Check sheet for the modelled part. Datum: model origin and axes. Units: mm. A direction names the side the tool comes from. Coordinates: 2 decimals unless noted, no trailing zeros. Order: outer loops, then holes, each group sorted by start corner. A loop starts at its lowest first (then second) coordinate and runs counter-clockwise, first axis right, second up.
1. Cross-section at C-C (z = -6.5). Enter the section's corners in (x, y), then the cut area to 3 significant figures.
2. Set-up check for faces 1 (the flat face through (4, -50.8, -12)), 2 (the cylindrical face through (20.111, -45.772, 2.948)), 3 (the flat face through (23.092, -25.578, 0.771)): record each of +Z, -Z, +X, -X, +Y, -Y from which the full face is reachable in a straight line by a thin tool's end or side.
3. Cross-section at D-D (x = -6.5). Enter the section's corners in (y, z).
4. Gauge pin test, flat ends, axial feed: pin 1 Ø1 at (y, z) = (-19, -19) entering from +X; pin 2 Ø8 at (x, z) = (-4.5, -14) entering from -Y; pin 3 Ø4 at (x, y) = (-6.5, -40.5) entering from -Z; pin 4 Ø8 at (x, y) = (-7, -8) entering from +Z. Record the tip position at first contact, or that the pin passes through.
5. Draft check along X on faces 4 (the cylindrical face through (23.46, -25.76, -40.04)), 5 (the cylindrical face through (21.862, -11.113, -0.215)), 6 (the cylindrical face through (19.072, -25.756, -38.868)). Enter one of: released by +X, released by -X, zero draft, split by the parting line, or undercut.
6. Thickness scan on line 1 (Y direction, x = 22, z = 1); line 2 (Z direction, x = 23.5, y = -30); line 3 (Z direction, x = 17, y = -42). Record the ranges inside material, lowest first.
7. Cross-section at A-A (y = -26). Count the separate pieces of the cut face and the enclosed holes in it, then the cut area to 3 significant figures.
```python
from build123d import *

# Parameters (mm, degrees)
F1_DEPTH = 50.8
F2_R     = 3.17499
F4_DEPTH = 25.4
F6_DEPTH = 25.4
F7_R     = 50.8
F8_DEPTH = 50.8
F9_R     = 3.175


# Not quite as in the source:
# - a fillet or chamfer is up to 0.001 mm smaller than in the source, because OpenCascade refuses the exact size
# - a feature names something its author has since deleted; it is built from what else it names


with BuildPart() as f1:
    # F0 (on Front) → F1 (new body)
    with BuildSketch(Plane.XZ):
        with BuildLine():
            ThreePointArc((24.0096036311, -41.4286058918), (25.0654524906, -37.313693309), (25.4207147422, -33.0803599757))
            ThreePointArc((25.4207147422, -33.0803599757), (24.2437436495, -25.4380520418), (20.821906037, -18.5039941488))
            Line((20.821906037, -18.5039941488), (20.1693195051, -17.2969153494))
            ThreePointArc((20.1693195051, -17.2969153494), (20.4643815884, -7.4727541905), (27.4307736322, -0.5394587257))
            Line((27.4307736322, -0.5394587257), (24.3787300207, 5.0289817915))
            ThreePointArc((24.3787300207, 5.0289817915), (22.9739817859, 4.2874085483), (21.5467011146, 3.5901866586))
            ThreePointArc((21.5467011146, 3.5901866586), (20.0925256969, 2.935513576), (18.6184879198, 2.3268793492))
            ThreePointArc((18.6184879198, 2.3268793492), (0, -1.2138607271), (-18.6184879198, 2.3268793492))
            ThreePointArc((-18.6184879198, 2.3268793492), (-20.0925256969, 2.935513576), (-21.5467011146, 3.5901866586))
            ThreePointArc((-21.5467011146, 3.5901866586), (-22.97860176, 4.289755995), (-24.3878181692, 5.0339641827))
            Line((-24.3878181692, 5.0339641827), (-27.4450352449, -0.5316376492))
            ThreePointArc((-27.4450352449, -0.5316376492), (-13.4987465328, -10.3152085141), (3.0701766945, -14.276017876))
            ThreePointArc((3.0701766945, -14.276017876), (14.5292424103, -20.7351129184), (19.0707147422, -33.0803599757))
            ThreePointArc((19.0707147422, -33.0803599757), (18.8042680535, -36.2553599757), (18.0123814088, -39.3415444128))
            Line((18.0123814088, -39.3415444128), (24.0096036311, -41.4286058918))
        make_face()
        with BuildLine():
            ThreePointArc((18.6184879198, 2.3268793492), (20.0925256969, 2.935513576), (21.5467011146, 3.5901866586))
            Line((21.5467011146, 3.5901866586), (19.869957668, 6.6493979065))
            Line((19.869957668, 6.6493979065), (17.0857374094, 5.1233761008))
            Line((17.0857374094, 5.1233761008), (18.6184879198, 2.3268793492))
        make_face()
        with BuildLine():
            ThreePointArc((-21.5467011146, 3.5901866586), (-20.0925256969, 2.935513576), (-18.6184879198, 2.3268793492))
            Line((-18.6184879198, 2.3268793492), (-17.0857374094, 5.1233761008))
            Line((-17.0857374094, 5.1233761008), (-19.869957668, 6.6493979065))
            Line((-19.869957668, 6.6493979065), (-21.5467011146, 3.5901866586))
        make_face()
    extrude(amount=F1_DEPTH)

    # F2 (radius 3.175 in the source; OpenCascade refuses exactly that, so slightly less here)
    f2_edges = [f1.edges().sort_by_distance(p)[0] for p in [
        (24.009604, -25.4, -41.428606),
        (18.012381, -25.4, -39.341544),
    ]]
    fillet(f2_edges, radius=F2_R)

    # F3 (on face) → F4 (cut)
    with BuildSketch(Plane(origin=(1.7876055886, 0, -3.2614787517), x_dir=(0.8769197665, 0, 0.4806367892), z_dir=(-0.4806367892, 0, 0.8769197665))):
        with BuildLine():
            Line((20.6203038983, -38.1), (20.6203038983, -12.7))
            ThreePointArc((20.6203038983, -12.7), (19.0328038983, -11.1125), (17.4453038983, -12.7))
            Line((17.4453038983, -12.7), (17.4453038983, -38.1))
            ThreePointArc((17.4453038983, -38.1), (19.0328038983, -39.6875), (20.6203038983, -38.1))
        make_face()
    extrude(amount=-F4_DEPTH, mode=Mode.SUBTRACT)

    # F5 (on face) → F6 (cut)
    with BuildSketch(Plane(origin=(-1.7876055886, 0, -3.2614787517), x_dir=(0.8769197665, 0, -0.4806367892), z_dir=(0.4806367892, 0, 0.8769197665))):
        with BuildLine():
            ThreePointArc((-20.6203038983, -38.1), (-19.0328038983, -39.6875), (-17.4453038983, -38.1))
            Line((-17.4453038983, -38.1), (-17.4453038983, -12.7))
            ThreePointArc((-17.4453038983, -12.7), (-19.0328038983, -11.1125), (-20.6203038983, -12.7))
            Line((-20.6203038983, -12.7), (-20.6203038983, -38.1))
        make_face()
    extrude(amount=-F6_DEPTH, mode=Mode.SUBTRACT)

    # F7 (on face) → F8 (cut)
    with BuildSketch(Plane(origin=(0, 0, 0), x_dir=(-1, 0, 0), z_dir=(0, 1, 0))):
        with Locations((-9.1173e-06, 49.5971090476)):
            Circle(F7_R)
    extrude(amount=-F8_DEPTH, mode=Mode.SUBTRACT)

    # F9
    f9_edges = [f1.edges().sort_by_distance(p)[0] for p in [
        (24.37873, -25.4, 5.028982),
        (27.430774, -25.4, -0.539459),
        (-24.387818, -25.4, 5.033964),
        (-27.445035, -25.4, -0.531638),
    ]]
    fillet(f9_edges, radius=F9_R)


solid = f1.part
```
Data:
1. outline: (-20.33, -50.8) - (20.93, -50.8) - (20.93, 0) - (-20.33, 0) - close
1. area: 2,100 mm2
2. face 1: +Z, -Z, +X, -X, -Y
2. face 2: +Z, +Y, -Y
2. face 3: none
3. outline: (-50.8, -12.8) - (0, -12.8) - (0, -0.8) - (-50.8, -0.8) - close
4. pin 1: stops at x = 21.49
4. pin 2: stops at y = -50.8
4. pin 3: stops at z = -13.28
4. pin 4: stops at z = -0.01
5. face 4: split by the parting line
5. face 5: undercut
5. face 6: released by -X
6. line 1: y = -50.8 to -39.5, -11.3 to 0
6. line 2: z = -40.02 to -23.39, 0.03 to 3.95
6. line 3: z = -24.44 to 1.72
7. separate pieces: 3
7. enclosed holes: 0
7. area: 753 mm2
